Check sheet for the drawn part. Datum: minimum x, y, z corner. Units: mm. A direction names the side the tool comes from. Round coordinates to 2 decimals unless told otherwise and drop trailing zeros. Order: outer loops, then holes, each group sorted by start corner. A loop starts at its lowest first (then second) coordinate and runs counter-clockwise, first axis right, second up. Notation, with made-up numbers: (1.25, 47.25) -> (54.25, 47.25) arc R15 cw to (54.25, 62.25) -> close; hole circle Ø6 at (-14.5, -19). An arc over 180 degrees is marked (long way). Answer as a JSON object with one key per item and string values. Group by question number.
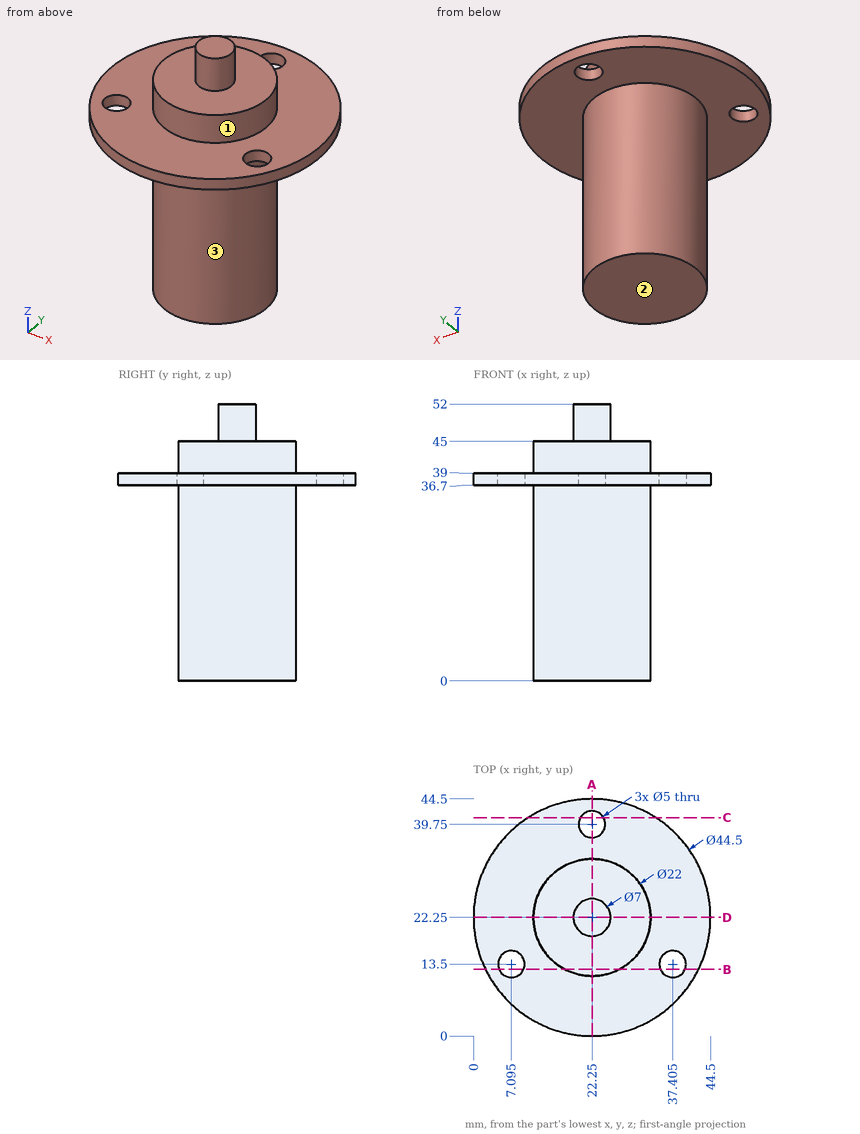
Item 1: Sectioned sample at C-C, the plane y = 41. Enter the section's corners in (x, z) (1 decimal).
Item 2: Depth check by flat-ended pin: pin 1 Ø6.5 at (x, y) = (22.25, 39.75) entering from +Z; pin 2 Ø5 at (x, z) = (24.5, 44) entering from -Y; pin 3 Ø1.5 at (y, z) = (29.5, 5.5) entering from -X (1 decimal). Enter the tip coordinate at first touch or a pass-through.
Item 3: Sectioned sample at A-A, the plane x = 22.25. Enter the section's corners in (y, z).
Item 4: Sectioned sample at B-B, the plane y = 12.5. Enter the section's corners in (x, z).
Item 5: Sectioned sample at D-D, the plane y = 22.25. Enter the section's corners in (x, z).
Item 6: Thickness scan on L1, parallel to X at y = 13, z = 37 (1 decimal); L2, parallel to Y at x = 22.25, z = 37.9; L3, parallel to Z at x = 10.5, y = 39. Record the ranges inside material, lowest first.
Item 7: Set-up check for the marked faces 1, 2 and 3: record each of +Z, -Z, +X, -X, +Y, -Y from which the full face is reachable in a straight line by a thin tool's end or side.
Result:
{
 "1": {"outline": "(10.3, 36.7) -> (20.1, 36.7) -> (20.1, 39) -> (10.3, 39) -> close; (24.4, 36.7) -> (34.2, 36.7) -> (34.2, 39) -> (24.4, 39) -> close"},
 "2": {"pin 1": "stops at z = 39", "pin 2": "stops at y = 11.25", "pin 3": "stops at x = 13.4"},
 "3": {"outline": "(0, 36.7) -> (11.25, 36.7) -> (11.25, 0) -> (33.25, 0) -> (33.25, 36.7) -> (37.25, 36.7) -> (37.25, 39) -> (33.25, 39) -> (33.25, 45) -> (25.75, 45) -> (25.75, 52) -> (18.75, 52) -> (18.75, 45) -> (11.25, 45) -> (11.25, 39) -> (0, 39) -> close; (42.25, 36.7) -> (44.5, 36.7) -> (44.5, 39) -> (42.25, 39) -> close"},
 "4": {"outline": "(2.25, 36.7) -> (4.8, 36.7) -> (4.8, 39) -> (2.25, 39) -> close; (9.39, 36.7) -> (17.16, 36.7) -> (17.16, 0) -> (27.34, 0) -> (27.34, 36.7) -> (35.11, 36.7) -> (35.11, 39) -> (27.34, 39) -> (27.34, 45) -> (17.16, 45) -> (17.16, 39) -> (9.39, 39) -> close; (39.7, 36.7) -> (42.25, 36.7) -> (42.25, 39) -> (39.7, 39) -> close"},
 "5": {"outline": "(0, 36.7) -> (11.25, 36.7) -> (11.25, 0) -> (33.25, 0) -> (33.25, 36.7) -> (44.5, 36.7) -> (44.5, 39) -> (33.25, 39) -> (33.25, 45) -> (25.75, 45) -> (25.75, 52) -> (18.75, 52) -> (18.75, 45) -> (11.25, 45) -> (11.25, 39) -> (0, 39) -> close"},
 "6": {"L1": "x = 2 to 4.6, 9.5 to 35, 39.9 to 42.5", "L2": "y = 0 to 37.25, 42.25 to 44.5", "L3": "z = 36.7 to 39"},
 "7": {"face 1": "+Z", "face 2": "-Z, +X, -X, +Y, -Y", "face 3": "-Z"}
}
